The listing builds one solid part. Answer for the finished solid, in the listing's coordinates (mm). A direction names the side the tool comes from. Round coordinates to 2 decimals unless told otherwise and drop trailing zeros. Write each loop counter-clockwise with the first axis right and the second up, starting at its lowest first coordinate (ties: lowest second). Pieces come first, ordered by that corner, then holes. Notation, with made-up numbers: (30, 49.25) - (84, 49.25) arc R17 ccw to (84, 79.25) - close; hole circle Ø2 at (-38, 9.25). An arc over 180 degrees is marked (long way). Return JSON: item names as keys, results as strings. Group by question number.
(1) Section B-B, the plane x = 0 is taken. Write down the section's boundary in (y, z).
(2) Each of these flat-tipped pins is pushed along its axis until it touches: pin 1 (3 mm diameter, centred on x = -10, z = 4, fed in from -Y); pin 2 (1.9 mm diameter, centred on y = -42, z = 2, fed in from -X). Where does it stop, or does it pass through?
(3) Find the intervals of material crossed by line 1 along Y through (x, z) = (-9.75, 3); line 2 along Y through (x, z) = (-0.25, 1); line 3 along X through (y, z) = (-26, 2), in increasing order. Write a range as [from, to].
(4) Section D-D, the plane y = 39 is taken. Write down the section's boundary in (x, z).
(5) Which of the six approach directions +Z, -Z, +X, -X, +Y, -Y give full straight-line access (tool end or side, diameter ignored) to faces 5 (the flat face through (6.35, 41, 3)), 6 (the flat face through (6.35, -41, 3)), 7 (the flat face through (-6.35, 41, 3))?
(6) Determine the mould class of faces 1 (the flat face through (0, 44.45, 3)), 2 (the flat face through (-12.7, -1, 3)), 3 (the cylindrical face through (-0.867, -29.305, 3.219)), 4 (the flat face through (9, -38.1, 3)) for opening direction Y: +Y half, -Y half, draft (parallel to the pull), parting line (faces both ways), or undercut.
(7) Section C-C, the plane z = 3.75 is taken. Write down the section's boundary in (x, y).
(8) Section A-A, the plane y = -25.4 is taken. Write down the section's boundary in (x, z).
```python
from build123d import *

# Parameters (mm, degrees)
SKETCH1_W           = 25.4
SKETCH1_H           = 76.2
SKETCH1_W_2         = 12.7
SKETCH1_H_2         = 6.35
BOSS_EXTRUDE1_DEPTH = 6.35
SKETCH2_R           = 4
CUT_EXTRUDE1_DEPTH  = 47.6627796


with BuildPart() as part:
    # Sketch1 → Boss-Extrude1 (new body)
    with BuildSketch(Plane.XY):
        Rectangle(SKETCH1_W, SKETCH1_H)
        with Locations((0, -41.275)):
            Rectangle(SKETCH1_W_2, SKETCH1_H_2)
        with Locations((0, 41.275)):
            Rectangle(SKETCH1_W_2, SKETCH1_H_2)
    extrude(amount=BOSS_EXTRUDE1_DEPTH)

    # Sketch2 → Cut-Extrude1 (cut, through all)
    with BuildSketch(Plane.XY.offset(6.35)):
        with Locations((0, -25.4)):
            Circle(SKETCH2_R)
    extrude(amount=-CUT_EXTRUDE1_DEPTH, mode=Mode.SUBTRACT)


solid = part.part
```
Working result:
{
 "1": {"outline": "(-44.45, 0) - (-29.4, 0) - (-29.4, 6.35) - (-44.45, 6.35) - close; (-21.4, 0) - (44.45, 0) - (44.45, 6.35) - (-21.4, 6.35) - close"},
 "2": {"pin 1": "stops at y = -38.1", "pin 2": "stops at x = -6.35"},
 "3": {"line 1": "y = [-38.1, 38.1]", "line 2": "y = [-44.45, -29.39], [-21.41, 44.45]", "line 3": "x = [-12.7, -3.95], [3.95, 12.7]"},
 "4": {"outline": "(-6.35, 0) - (6.35, 0) - (6.35, 6.35) - (-6.35, 6.35) - close"},
 "5": {"face 5": "+Z, -Z, +X, +Y", "face 6": "+Z, -Z, +X, -Y", "face 7": "+Z, -Z, -X, +Y"},
 "6": {"face 1": "+Y half", "face 2": "draft", "face 3": "undercut", "face 4": "-Y half"},
 "7": {"outline": "(-12.7, -38.1) - (-6.35, -38.1) - (-6.35, -44.45) - (6.35, -44.45) - (6.35, -38.1) - (12.7, -38.1) - (12.7, 38.1) - (6.35, 38.1) - (6.35, 44.45) - (-6.35, 44.45) - (-6.35, 38.1) - (-12.7, 38.1) - close; hole circle Ø8 at (0, -25.4)"},
 "8": {"outline": "(-12.7, 0) - (-4, 0) - (-4, 6.35) - (-12.7, 6.35) - close; (4, 0) - (12.7, 0) - (12.7, 6.35) - (4, 6.35) - close"}
}
